```python
from build123d import *

# Parameters (mm, degrees)
SKETCH1_R           = 8.5
SKETCH1_R_2         = 4.6
BOSS_EXTRUDE1_DEPTH = 5.75
BOSS_EXTRUDE2_START = 1.5
SKETCH2_R           = 8.5
SKETCH2_R_2         = 7.1
BOSS_EXTRUDE2_DEPTH = 1.5
SKETCH3_R           = 8.5
SKETCH3_R_2         = 4
BOSS_EXTRUDE3_DEPTH = 1
SKETCH4_R           = 6.65
SKETCH4_R_2         = 5.45
BOSS_EXTRUDE4_DEPTH = 1.5
BOSS_EXTRUDE5_START = -8.25
SKETCH5_R           = 7.1
BOSS_EXTRUDE5_DEPTH = 8.25
FILLET1_SIZE        = 3
SKETCH6_R           = 1.575
CUT_EXTRUDE1_DEPTH  = 1.8
SKETCH6_3_R         = 1.575
CUT_EXTRUDE2_DEPTH  = 23.804878934
SHELL1_START        = 2
SHELL1_DEPTH        = 2.75
SHELL1_START_2      = 0.5
SHELL1_2_DEPTH      = 1.5


with BuildPart() as part:
    # Sketch1 → Boss-Extrude1 (new body)
    with BuildSketch(Plane.XY):
        Circle(SKETCH1_R)
        Circle(SKETCH1_R_2, mode=Mode.SUBTRACT)
    extrude(amount=BOSS_EXTRUDE1_DEPTH)

    # Sketch2 → Boss-Extrude2 (add)
    with BuildSketch(Plane(origin=(0, 0, 0), x_dir=(-1, 0, 0), z_dir=(0, 0, -1)).offset(BOSS_EXTRUDE2_START)):
        Circle(SKETCH2_R)
        Circle(SKETCH2_R_2, mode=Mode.SUBTRACT)
    extrude(amount=-BOSS_EXTRUDE2_DEPTH)

    # Sketch3 → Boss-Extrude3 (add)
    with BuildSketch(Plane.XY.offset(5.75)):
        with Locations(Location((0, 0, 0), (0, 0, 180))):
            Circle(SKETCH3_R)
        Circle(SKETCH3_R_2, mode=Mode.SUBTRACT)
    extrude(amount=BOSS_EXTRUDE3_DEPTH)

    # Sketch4 → Boss-Extrude4 (add)
    with BuildSketch(Plane.XY.offset(6.75)):
        Circle(SKETCH4_R)
        Circle(SKETCH4_R_2, mode=Mode.SUBTRACT)
    extrude(amount=BOSS_EXTRUDE4_DEPTH)

    # Sketch5 → Boss-Extrude5 (add)
    with BuildSketch(Plane.XY.offset(6.75).offset(BOSS_EXTRUDE5_START)):
        with BuildLine():
            Line((-8.5, 0), (-8.5, -5.5))
            Line((-8.5, -5.5), (-16, -5.5))
            Line((-16, -5.5), (-16, -8.5))
            Line((-16, -8.5), (16, -8.5))
            Line((16, -8.5), (16, -5.5))
            Line((16, -5.5), (8.5, -5.5))
            Line((8.5, -5.5), (8.5, 0))
            ThreePointArc((8.5, 0), (0, 8.5), (-8.5, 0))
        make_face()
        with Locations(Location((0, 0, 0), (0, 0, 180))):
            Circle(SKETCH5_R, mode=Mode.SUBTRACT)
    extrude(amount=BOSS_EXTRUDE5_DEPTH)

    # Fillet1
    # a fillet whose section is not a circle: 3 mm, written as the material it takes off along each edge
    with BuildSketch(Plane(origin=(-16, 2, -1.5), x_dir=(0, 0, 1), z_dir=(0, -1, 0)), Plane(origin=(-16, 2, 6.75), x_dir=(1, 0, 0), z_dir=(0, -1, 0)), Plane(origin=(16, -16, -1.5), x_dir=(0, 0, 1), z_dir=(0, 1, 0)), Plane(origin=(16, -16, 6.75), x_dir=(-1, 0, 0), z_dir=(0, 1, 0))) as fillet1_piece_1:
        with BuildLine():
            add(Edge.make_bspline([(FILLET1_SIZE, 0), (FILLET1_SIZE * 0.831801948466, 0), (FILLET1_SIZE * 0.663603896932, 0), (FILLET1_SIZE * 0.292893218813, -FILLET1_SIZE * 0.0716919198361), (FILLET1_SIZE * 0.0716919198361, -FILLET1_SIZE * 0.292893218813), (0, -FILLET1_SIZE * 0.663603896932), (0, -FILLET1_SIZE * 0.831801948466), (0, -FILLET1_SIZE)], knots=[0, 0, 0, 0, 0, 0, 0.5, 0.5, 1, 1, 1, 1, 1, 1], degree=5))
            Line((0, -FILLET1_SIZE), (0, 0))
            Line((0, 0), (FILLET1_SIZE, 0))
        make_face()
    extrude(amount=18, mode=Mode.SUBTRACT)

    # Sketch6 → Cut-Extrude1 (cut)
    # profile 1 of 2: a face of its own
    with BuildSketch(Plane(origin=(0, -5.5, 0), x_dir=(1, 0, 0), z_dir=(0, 1, 0))):
        Polygon((-11.35, 0.665896534), (-14.2, -0.979551733), (-14.2, -4.270448267), (-11.35, -5.915896534), (-8.5, -4.270448267), (-8.5, -0.979551733), align=None)
        with Locations((-11.35, -2.625)):
            Circle(SKETCH6_R, mode=Mode.SUBTRACT)
    # profile 2 of 2: a face of its own
    with BuildSketch(Plane(origin=(0, -5.5, 0), x_dir=(1, 0, 0), z_dir=(0, 1, 0))):
        with Locations((-11.35, -2.625)):
            Circle(SKETCH6_R)
    cut_extrude1 = extrude(amount=-CUT_EXTRUDE1_DEPTH, mode=Mode.SUBTRACT)

    # Sketch6<3> → Cut-Extrude2 (cut, through all)
    with BuildSketch(Plane(origin=(0, -5.5, 0), x_dir=(1, 0, 0), z_dir=(0, 1, 0))):
        with Locations(Location((-11.35, -2.625, 0), (0, 0, 270))):
            Circle(SKETCH6_3_R)
    cut_extrude2 = extrude(amount=-CUT_EXTRUDE2_DEPTH, mode=Mode.SUBTRACT)

    # Mirror1: Cut-Extrude1, Cut-Extrude2 across plane
    add(cut_extrude1.mirror(Plane(origin=(0, 0, 0), x_dir=(0, 0, 1), z_dir=(1, 0, 0))), mode=Mode.SUBTRACT)
    add(cut_extrude2.mirror(Plane(origin=(0, 0, 0), x_dir=(0, 0, 1), z_dir=(1, 0, 0))), mode=Mode.SUBTRACT)

    # Shell1: read off the stored shape, not the designer's step
    # Shell1 outline → Shell1 (cut)
    with BuildSketch(Plane.XY.offset(SHELL1_START)):
        with BuildLine():
            ThreePointArc((6.5, -1.144552314), (0, -6.6), (-6.5, -1.144552314))
            Line((-6.5, -1.144552314), (-6.5, -8.5))
            Line((-6.5, -8.5), (6.5, -8.5))
            Line((6.5, -8.5), (6.5, -1.144552314))
        make_face()
    extrude(amount=SHELL1_DEPTH, mode=Mode.SUBTRACT)

    # Shell1 2 outline → Shell1 2 (cut)
    with BuildSketch(Plane.XY.offset(SHELL1_START_2)):
        with BuildLine():
            Line((6.5, -8.5), (6.5, -6.368673331))
            ThreePointArc((6.5, -6.368673331), (4.989928684, -7.609902216), (3.249615362, -8.5))
            Line((3.249615362, -8.5), (6.5, -8.5))
        make_face()
        with BuildLine():
            ThreePointArc((-3.249615362, -8.5), (-4.989928684, -7.609902216), (-6.5, -6.368673331))
            Line((-6.5, -6.368673331), (-6.5, -8.5))
            Line((-6.5, -8.5), (-3.249615362, -8.5))
        make_face()
    extrude(amount=SHELL1_2_DEPTH, mode=Mode.SUBTRACT)


solid = part.part
```
Design review of the part built by this model. Coordinates are the model's own, in mm. A direction names the side the tool comes from. Give positions to 0.01 mm unless a question says otherwise; leave off trailing zeros. Order: outer loops, then holes, each group sorted by start corner. A loop starts at its lowest first (then second) coordinate and runs counter-clockwise, first axis right, second up. Notation, with made-up numbers: (-18, -9) -> (37, -9) arc R23 ccw to (37, 17) -> close; hole circle Ø9 at (-14, 52.5). An arc over 180 degrees is marked (long way). Write item = value, one per line. Start each with the question number.
(1) We need section A-A on y = -2.25. State how many separate pieces and enclosed holes the cut face has, plus the area to 3 significant figures.
(2) We need section B-B on y = 1.25. Write out the cut boundary in (x, z).
(3) Mouldability with a two-part tool opening along Y and no side actions: class faces 1 (the face through (0, -7, 4.75)), 2 (the face through (-15, -5.5, 3)), 3 (the face through (0.92, 7.04, -0.76)) as +Y half, -Y half, draft (parallel to the pull), parting line (faces both ways), or undercut.
(4) For pin 1 (2 mm diameter, centred on y = -4, z = 3, fed in from -X); pin 2 (4.5 mm diameter, centred on x = 1.5, y = -2, fed in from +Z); pin 3 (2.5 mm diameter, centred on x = 11, z = 2, fed in from +Y); pin 4 (6.5 mm diameter, centred on x = 0, y = 0, fed in from -Z), all flat-tipped, find the tip position at first contact; note any pin that passes through.
(5) To check wall thickness, follow line 1 along Z through (x, y) = (11.35, -7.9); line 2 along Y through (x, z) = (0, 1.3); line 3 along Y through (x, z) = (0, -0.55). State the ranges of each line that lie inside material, in increasing order.
(6) We need section D-D on x = -7.5. Write out the cut boundary in (y, z), plus the area to 3 significant figures.
(7) For faces 4 (the face through (2, -4, 6.75)), 5 (the face through (12.76, -6.39, 0.15)), 6 (the face through (6, -8, 0.5)), 7 (the face through (15, -5.5, 3)), list the 3-axis set-ups (+Z, -Z, +X, -X, +Y, -Y) from which the entire face can be reached by the end or side of a thin tool; tool diameter is ignored.
(8) We need section C-C on y = -5. Write out the cut boundary in (x, z).
Numbers:
q1.separate_pieces = 2
q1.enclosed_holes = 2
q1.area = 69.6 mm^2
q2.outline = (-8.41, -1.5) -> (-6.99, -1.5) -> (-6.99, 0) -> (-4.43, 0) -> (-4.43, 5.75) -> (-3.8, 5.75) -> (-3.8, 6.75) -> (-5.3, 6.75) -> (-5.3, 8.25) -> (-6.53, 8.25) -> (-6.53, 6.75) -> (-8.41, 6.75) -> close; (3.8, 5.75) -> (4.43, 5.75) -> (4.43, 0) -> (6.99, 0) -> (6.99, -1.5) -> (8.41, -1.5) -> (8.41, 6.75) -> (6.53, 6.75) -> (6.53, 8.25) -> (5.3, 8.25) -> (5.3, 6.75) -> (3.8, 6.75) -> close
q3.face_1 = draft
q3.face_2 = +Y half
q3.face_3 = undercut
q4.pin_1 = -8.5
q4.pin_2 = 6.75
q4.pin_3 = -7.3
q4.pin_4 = through
q5.line_1 = -1.5 to 1.05, 4.2 to 6.75
q5.line_2 = -8.5 to -4.6, 4.6 to 8.5
q5.line_3 = -8.5 to -7.1, 7.1 to 8.5
q6.outline = (-8.5, -1.5) -> (4, -1.5) -> (4, 6.75) -> (-8.5, 6.75) -> close
q6.area = 103 mm^2
q7.face_4 = +Z
q7.face_5 = +Y
q7.face_6 = -Y
q7.face_7 = +Z, -Z, +X, +Y
q8.outline = (-8.5, -1.5) -> (-5.04, -1.5) -> (-5.04, 0) -> (5.04, 0) -> (5.04, -1.5) -> (8.5, -1.5) -> (8.5, 6.75) -> (4.38, 6.75) -> (4.38, 8.25) -> (2.17, 8.25) -> (2.17, 6.75) -> (-2.17, 6.75) -> (-2.17, 8.25) -> (-4.38, 8.25) -> (-4.38, 6.75) -> (-8.5, 6.75) -> close; hole (-6.5, 2) -> (-4.31, 2) -> (-4.31, 4.75) -> (-6.5, 4.75) -> close; hole (4.31, 2) -> (6.5, 2) -> (6.5, 4.75) -> (4.31, 4.75) -> close
